Could you check a few things on this model? Use its own coordinates, in mm. Face numbers are marked on the shaded views. Coordinates: 2 decimals unless noted, no trailing zeros. Loops run counter-clockwise (first coordinate to the right, second up) from the corner with the lowest first, then second, coordinate; pieces in that order, holes last. Notation, with made-up numbers: (-4, -25) - (41, -25) arc R24 cw to (41, -6) - close; hole circle Ø7 at (-11.75, 61). An arc over 180 degrees is marked (long way). One line per question, with ' | ' between items. Start each with the question number.
1. I'm going to push flat-ended pins straight in: P1, Ø8, axis at y = 25.5, z = -14.5, coming from the -X side; P2, Ø6, axis at y = 10, z = -6.5, coming from the -X side; P3, Ø5, axis at y = 25.5, z = -10, coming from the -X side. Where does each tip first touch, or does it pass through?
2. We'd pull the mould along X, two halves only. Please class the marked faces 1, 2 and 3: pulls with the +X half, pulls with the -X half, needs draft (parallel to the pull), parting line crosses it, or undercut.
3. I want a section at B-B, the plane x = 0. Write out the boundary of the cut face in (y, z), then the cut area to 3 significant figures.
4. I want a section at C-C, the plane z = 0. Write out the boundary of the cut face in (x, y), then the cut area to 3 significant figures.
5. I want a section at D-D, the plane y = 13.5. Write out the boundary of the cut face in (x, z), then the cut area to 3 significant figures.
6. I want a section at A-A, the plane y = 45. Write out the boundary of the cut face in (x, z), then the cut area to 3 significant figures.
7. Please list where these lines run through material, in increasing order: L1, parallel to X at y = 43, z = 0; L2, parallel to Y at x = 4.5, z = -16. Write a range as [from, to].
Autodesk Inventor part; units mm, degrees
ref_plane "YZ Plane" through (0, 0, 0) normal (1, 0, 0) x (0, 1, 0)
ref_plane "XZ Plane" through (0, 0, 0) normal (0, 1, 0) x (-1, 0, 0)
ref_plane "XY Plane" through (0, 0, 0) normal (0, 0, 1) x (1, 0, 0)
sketch "Sketch30" plane through (0, 0, 0) normal (0, 1, 0) x (-1, 0, 0)
  circle A0 centre (0, 0) radius 25
  dimension "d117" = 50
extrude "Extrusion21" add sketch "Sketch30" along normal blind 30
sketch "Sketch31" plane through (0, 30, 0) normal (0, 1, 0) x (1, 0, 0)
  circle A0 centre (0, 0) radius 15
  dimension "d120" = 30
extrude "Extrusion22" add sketch "Sketch31" along normal blind 30
sketch "Sketch32" plane through (0, 60, 0) normal (0, 1, 0) x (1, 0, 0)
  circle A0 centre (0, 0) radius 15
  circle A1 centre (0, 0) radius 12.5
  dimension "d123" = 25
extrude "Extrusion23" cut sketch "Sketch32" against normal blind 30 contours A1
sketch "Sketch33" plane through (0, 0, 0) normal (0, -1, 0) x (1, 0, 0)
  point P0 (0, 0)
properties part number "Front_base"
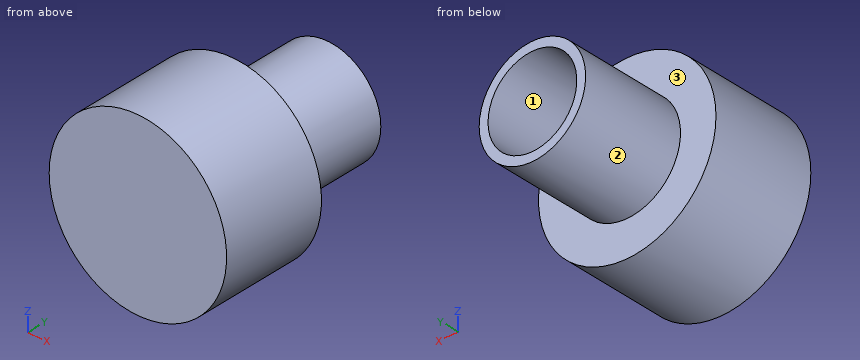
Results are:
1) P1: stops at x = -22.69 | P2: stops at x = -24.75 | P3: stops at x = -23.85
2) face 1: undercut | face 2: parting line crosses it | face 3: needs draft
3) outline: (0, -25) - (30, -25) - (30, -15) - (60, -15) - (60, -12.5) - (30, -12.5) - (30, 12.5) - (60, 12.5) - (60, 15) - (30, 15) - (30, 25) - (0, 25) - close | area: 1,650 mm2
4) outline: (-25, 0) - (25, 0) - (25, 30) - (15, 30) - (15, 60) - (12.5, 60) - (12.5, 30) - (-12.5, 30) - (-12.5, 60) - (-15, 60) - (-15, 30) - (-25, 30) - close | area: 1,650 mm2
5) outline: circle Ø50 at (0, 0) | area: 1,960 mm2
6) outline: circle Ø30 at (0, 0); hole circle Ø25 at (0, 0) | area: 216 mm2
7) L1: x = [-15, -12.5], [12.5, 15] | L2: y = [0, 30]
